Can you work these out from the model? Positions are in its coordinate system, mm. Round coordinates to 2 decimals unless told otherwise and drop trailing zeros. Order: outer loops, then holes, each group sorted by start corner. A loop starts at its lowest first (then second) coordinate and runs counter-clockwise, first axis right, second up.
Q1. If we section it at A-A (x = -14): Please give me the cut outline in (y, z).
Q2. If we section it at C-C (y = 18): Please give me the cut outline in (x, z).
Q3. If we section it at B-B (y = 2.5): Please give me the cut outline in (x, z).
Q4. If I drill on line 1 (Y direction, x = 13.5, z = 4.7); line 2 (X direction, y = 22, z = 4.2), over which ranges is the centre line in solid material (lowest first)?
from build123d import *

# Parameters (mm, degrees)
ESQUISSE1_W             = 82
ESQUISSE1_H             = 87
BOSS_EXTRU_1_DEPTH      = 5
ENL_V_MAT_EXTRU_1_DEPTH = 1


with BuildPart() as part:
    # Esquisse1 → Boss.-Extru.1 (new body)
    with BuildSketch(Plane.XY):
        Rectangle(ESQUISSE1_W, ESQUISSE1_H)
    extrude(amount=BOSS_EXTRU_1_DEPTH)

    # Esquisse2 → Enlèv. mat.-Extru.1 (cut)
    # profile 1 of 3: a face of its own
    with BuildSketch(Plane.XY.offset(5)):
        with BuildLine():
            Line((-30.820713327, 24.668633563), (-30.820713327, -6.212394271))
            Line((-30.820713327, -6.212394271), (-28.820713327, -6.212394271))
            Line((-28.820713327, -6.212394271), (-28.820713327, 22.838674714))
            ThreePointArc((-28.820713327, 22.838674714), (-20.675920897, 15.227477844), (-27.444134647, 6.369755555))
            Line((-27.444134647, 6.369755555), (-27.081213863, 4.402959047))
            ThreePointArc((-27.081213863, 4.402959047), (-18.818126337, 16.405546037), (-30.820713327, 24.668633563))
        make_face()
    # profile 2 of 3: a face of its own
    with BuildSketch(Plane.XY.offset(5)):
        with BuildLine():
            Line((-5.247362152, -6.212394271), (-4.768401098, -4.270591936))
            ThreePointArc((-4.768401098, -4.270591936), (-15.342116904, 9.228119646), (-4.768401098, 22.726831228))
            Line((-4.768401098, 22.726831228), (-5.247362152, 24.668633563))
            ThreePointArc((-5.247362152, 24.668633563), (-17.342116904, 9.228119646), (-5.247362152, -6.212394271))
        make_face()
    # profile 3 of 3: a face of its own
    with BuildSketch(Plane.XY.offset(5)):
        with BuildLine():
            Line((7.177426391, 24.753119096), (7.177426391, -5.822234801))
            ThreePointArc((7.177426391, -5.822234801), (15.465789743, -0.161602052), (13.20887714, 9.618279116))
            ThreePointArc((13.20887714, 9.618279116), (14.745705745, 18.999957145), (7.177426391, 24.753119096))
        make_face()
        with BuildLine():
            Line((9.177426391, 22.155705275), (9.177426391, -3.525944184))
            ThreePointArc((9.177426391, -3.525944184), (14.064473769, 2.682629125), (9.916217396, 9.407328648))
            ThreePointArc((9.916217396, 9.407328648), (13.388733311, 16.004162532), (9.177426391, 22.155705275))
        make_face(mode=Mode.SUBTRACT)
    extrude(amount=-ENL_V_MAT_EXTRU_1_DEPTH, mode=Mode.SUBTRACT)


solid = part.part
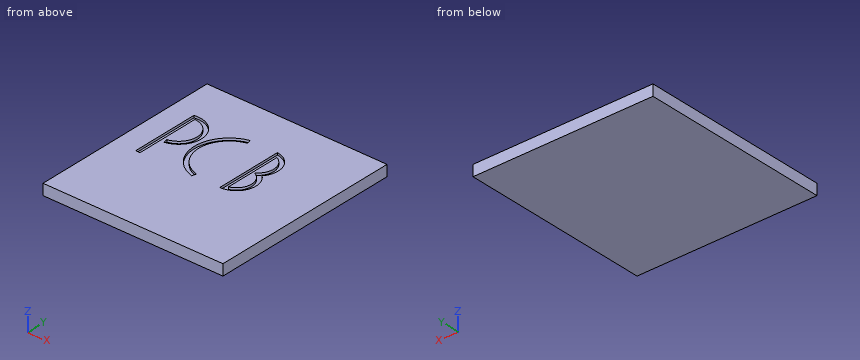
Solution:
1. outline: (-43.5, 0) - (43.5, 0) - (43.5, 5) - (18.98, 5) - (18.98, 4) - (15.19, 4) - (15.19, 5) - (3.27, 5) - (3.27, 4) - (-0.53, 4) - (-0.53, 5) - (-43.5, 5) - close
2. outline: (-41, 0) - (41, 0) - (41, 5) - (15.08, 5) - (15.08, 4) - (12.99, 4) - (12.99, 5) - (9.18, 5) - (9.18, 4) - (7.18, 4) - (7.18, 5) - (-12.23, 5) - (-12.23, 4) - (-14.7, 4) - (-14.7, 5) - (-19.25, 5) - (-19.25, 4) - (-21.4, 4) - (-21.4, 5) - (-28.82, 5) - (-28.82, 4) - (-30.82, 4) - (-30.82, 5) - (-41, 5) - close
3. outline: (-41, 0) - (41, 0) - (41, 5) - (16.06, 5) - (16.06, 4) - (14.05, 4) - (14.05, 5) - (9.18, 5) - (9.18, 4) - (7.18, 4) - (7.18, 5) - (-13.61, 5) - (-13.61, 4) - (-15.85, 4) - (-15.85, 5) - (-28.82, 5) - (-28.82, 4) - (-30.82, 4) - (-30.82, 5) - (-41, 5) - close
4. line 1: y = -43.5 to -3.19, 0.32 to 5.83, 9.34 to 9.98, 21.19 to 43.5
4. line 2: x = -41 to -30.82, -28.82 to -25.31, -21.85 to -10.91, -6.93 to 7.18, 9.18 to 9.5, 12.8 to 41
